Source: CAD feature listing. Evaluate the final solid. Frame: model axes, mm. Face numbers are marked on the shaded views. A direction names the side the tool comes from. Give positions to 0.01 mm unless a question says otherwise; leave off trailing zeros. Loops run counter-clockwise (first coordinate to the right, second up) from the corner with the lowest first, then second, coordinate; pieces in that order, holes last.
```python
from build123d import *

# Parameters (mm, degrees)
SKETCH_1_W          = 60
SKETCH_1_H          = 20
EXTRUDE_1_DEPTH     = 6
CUT_EXTRUDE_1_DEPTH = 6
SKETCH_3_R          = 5
CUT_EXTRUDE_2_DEPTH = 3
EXTRUDE_2_DEPTH     = 14
CUT_EXTRUDE_3_DEPTH = 20
SKETCH_6_W          = 20
SKETCH_6_H          = 20
EXTRUDE_3_DEPTH     = 14
SKETCH_7_W          = 20
SKETCH_7_H          = 20
EXTRUDE_4_DEPTH     = 54
SKETCH_8_W          = 15
SKETCH_8_H          = 15
CUT_EXTRUDE_4_DEPTH = 64
SKETCH_9_W          = 19.9
SKETCH_9_H          = 10.2
CUT_EXTRUDE_5_DEPTH = 17.5
SKETCH_11_W         = 19.9
SKETCH_11_H         = 10.2
CUT_EXTRUDE_6_DEPTH = 15
SKETCH_12_W         = 35.1
SKETCH_12_H         = 10.2
EXTRUDE_5_DEPTH     = 2.5
CUT_EXTRUDE_7_DEPTH = 2.5


with BuildPart() as part:
    # 草图1 → 凸台-拉伸1 (new body)
    with BuildSketch(Plane(origin=(0, 0, 0), x_dir=(1, 0, 0), z_dir=(0, 1, 0))):
        Rectangle(SKETCH_1_W, SKETCH_1_H)
    extrude(amount=EXTRUDE_1_DEPTH)

    # 草图2 → 切除-拉伸1 (cut)
    with BuildSketch(Plane(origin=(0, 6, 0), x_dir=(1, 0, 0), z_dir=(0, 1, 0))):
        with BuildLine():
            ThreePointArc((22.6, 0), (20, 2.6), (17.4, 0))
            Line((17.4, 0), (22.6, 0))
        make_face()
        with BuildLine():
            Line((22.6, 0), (17.4, 0))
            ThreePointArc((17.4, 0), (20, -2.6), (22.6, 0))
        make_face()
    extrude(amount=-CUT_EXTRUDE_1_DEPTH, mode=Mode.SUBTRACT)

    # 草图3 → 切除-拉伸2 (cut)
    with BuildSketch(Plane(origin=(0, 6, 0), x_dir=(1, 0, 0), z_dir=(0, 1, 0))):
        with Locations(Location((20, 0, 0), (0, 0, 270))):
            Circle(SKETCH_3_R)
    extrude(amount=-CUT_EXTRUDE_2_DEPTH, mode=Mode.SUBTRACT)

    # 草图4 → 凸台-拉伸2 (add)
    with BuildSketch(Plane(origin=(0, 6, 0), x_dir=(1, 0, 0), z_dir=(0, 1, 0))):
        Polygon((-10, -10), (0, -10), (10, -10), (10, 10), (0, 10), (-10, 10), align=None)
    extrude(amount=EXTRUDE_2_DEPTH)

    # 草图5 → 切除-拉伸3 (cut)
    with BuildSketch(Plane(origin=(0, 20, 0), x_dir=(1, 0, 0), z_dir=(0, 1, 0))):
        Polygon((-7.6, 0), (0, 0), (7.6, 0), (7.6, 5.1), (-7.6, 5.1), align=None)
        Polygon((7.6, 0), (0, 0), (-7.6, 0), (-7.6, -5.1), (7.6, -5.1), align=None)
    extrude(amount=-CUT_EXTRUDE_3_DEPTH, mode=Mode.SUBTRACT)

    # 草图6 → 凸台-拉伸3 (add)
    with BuildSketch(Plane(origin=(0, 6, 0), x_dir=(1, 0, 0), z_dir=(0, 1, 0))):
        with Locations((-20, 0)):
            Rectangle(SKETCH_6_W, SKETCH_6_H)
    extrude(amount=EXTRUDE_3_DEPTH)

    # 草图7 → 凸台-拉伸4 (add)
    with BuildSketch(Plane.XY.offset(10)):
        with Locations((-20, 10)):
            Rectangle(SKETCH_7_W, SKETCH_7_H)
    extrude(amount=EXTRUDE_4_DEPTH)

    # 草图8 → 切除-拉伸4 (cut)
    with BuildSketch(Plane.XY.offset(64)):
        with Locations((-20, 10)):
            Rectangle(SKETCH_8_W, SKETCH_8_H)
    extrude(amount=-CUT_EXTRUDE_4_DEPTH, mode=Mode.SUBTRACT)

    # 草图9 → 切除-拉伸5 (cut)
    with BuildSketch(Plane(origin=(0, 20, 0), x_dir=(1, 0, 0), z_dir=(0, 1, 0))):
        with Locations((-17.55, 0)):
            Rectangle(SKETCH_9_W, SKETCH_9_H)
    extrude(amount=-CUT_EXTRUDE_5_DEPTH, mode=Mode.SUBTRACT)

    # 草图11 → 切除-拉伸6 (cut)
    with BuildSketch(Plane(origin=(0, 2.5, 0), x_dir=(1, 0, 0), z_dir=(0, 1, 0))):
        with Locations((-17.55, 0)):
            Rectangle(SKETCH_11_W, SKETCH_11_H)
    extrude(amount=-CUT_EXTRUDE_6_DEPTH, mode=Mode.SUBTRACT)

    # 草图12 → 凸台-拉伸5 (add)
    with BuildSketch(Plane(origin=(0, 20, 0), x_dir=(1, 0, 0), z_dir=(0, 1, 0))):
        with Locations((-9.95, 0)):
            Rectangle(SKETCH_12_W, SKETCH_12_H)
    extrude(amount=-EXTRUDE_5_DEPTH)

    # 草图13 → 切除-拉伸7 (cut)
    with BuildSketch(Plane(origin=(0, 20, 0), x_dir=(1, 0, 0), z_dir=(0, 1, 0))):
        Polygon((-7.6, 0), (0, 0), (7.6, 0), (7.6, 5.1), (-7.6, 5.1), align=None)
        Polygon((7.6, 0), (0, 0), (-7.6, 0), (-7.6, -5.1), (7.6, -5.1), align=None)
    extrude(amount=-CUT_EXTRUDE_7_DEPTH, mode=Mode.SUBTRACT)


solid = part.part
```
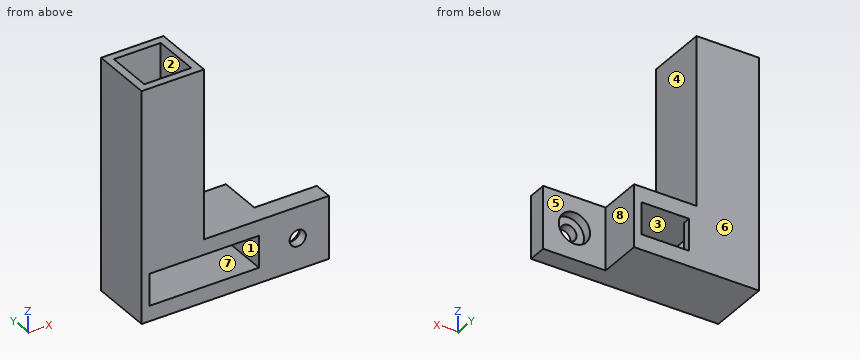
(1) Section C-C, the plane y = 5. Return the cut outline in (x, z), then the cut area to 3 significant figures.
A:
outline: (-30, -10) - (30, -10) - (30, 10) - (-10, 10) - (-10, 64) - (-12.5, 64) - (-12.5, 5.1) - (7.6, 5.1) - (7.6, -5.1) - (-27.5, -5.1) - (-27.5, 64) - (-30, 64) - close; hole circle Ø10 at (20, 0)
area: 960 mm2
(2) Section A-A, the plane x = -0.5. Return the cut outline in (y, z), then the cut area to 3 significant figures.
A:
outline: (0, -10) - (20, -10) - (20, -5.1) - (0, -5.1) - close; (0, 5.1) - (20, 5.1) - (20, 10) - (0, 10) - close
area: 196 mm2
(3) Ray query, line 1 along X through (y, z) = (3.9, 0); line 2 along X through (y, z) = (9.25, 4); line 3 along Z through (x, y) = (20, 1.45). Return the intervals inside material, ascending.
A:
line 1: x = -30 to -27.5, 7.6 to 15, 25 to 30
line 2: x = -30 to -27.5, 7.6 to 10
line 3: z = -10 to -2.6, 2.6 to 10
(4) Section D-D, the plane z = 34.5. Return the cut outline in (x, y), then the cut area to 3 significant figures.
A:
outline: (-30, 0) - (-10, 0) - (-10, 20) - (-30, 20) - close; hole (-27.5, 2.5) - (-12.5, 2.5) - (-12.5, 17.5) - (-27.5, 17.5) - close
area: 175 mm2
(5) Reachability of the marked faces 1, 2, 3, 4 and 5 from +Z, -Z, +X, -X, +Y, -Y: full face, straight path, thin tool, end or side. Return the list, or none.
A:
face 1: +Y, -Y
face 2: +Z
face 3: -Y
face 4: +Z, +X, +Y, -Y
face 5: +Z, -Z, +X, +Y
(6) First-contact query: pin 1 (10 mm diameter, centred on y = 3, z = 46.5, fed in from +X); pin 2 (7 mm diameter, centred on x = 20, z = 0, fed in from +Y); pin 3 (6 mm diameter, centred on x = -21, z = 42, fed in from -Y); pin 4 (5 mm diameter, centred on x = -1, y = 7, fed in from +Z). Flat tips, straight axial feed; report the tip coordinate or a pass-through.
A:
pin 1: stops at x = -10
pin 2: stops at y = 3
pin 3: stops at y = 0
pin 4: stops at z = 10
(7) Section B-B, the plane z = 0. Return the cut outline in (x, y).
A:
outline: (-30, 0) - (-27.5, 0) - (-27.5, 17.5) - (-7.6, 17.5) - (-7.6, 20) - (-30, 20) - close; (7.6, 0) - (17.4, 0) - (17.4, 3) - (15, 3) - (15, 6) - (10, 6) - (10, 20) - (7.6, 20) - close; (22.6, 0) - (30, 0) - (30, 6) - (25, 6) - (25, 3) - (22.6, 3) - close
(8) Mould query, pull axis X, two halves, no side actions, for the marked faces 6, 7 and 8. Classes: pulls with the +X half, pulls with the -X half, needs draft (parallel to the pull), parting line crosses it, or undercut.
A:
face 6: needs draft
face 7: undercut
face 8: pulls with the +X half
